from build123d import *

# Parameters (mm, degrees)
SKETCH_8_R          = 8
SKETCH_8_R_2        = 1.5
SKETCH_8_R_3        = 1.55
SKETCH_8_R_4        = 2.05
EXTRUDE_2522_DEPTH  = 3
FILLET_27_R         = 6
FILLET_30_R         = 3
FILLET_31_R         = 2
SKETCH_9_R          = 2.05
CUT_EXTRUDE_1_DEPTH = 172.249087589


with BuildPart() as part:
    # Эскиз8 → Extrude 2522 (new body)
    with BuildSketch(Plane.XY):
        with BuildLine():
            Line((38.676576093, 1), (169, 1))
            Line((169, 1), (169, -15))
            Line((169, -15), (90, -15))
            Line((90, -15), (12, -15))
            Line((12, -15), (10, -17))
            Line((10, -17), (4.230786919, -17))
            ThreePointArc((4.230786919, -17), (0, -17.231764199), (-4.230786919, -17))
            Line((-4.230786919, -17), (-10, -17))
            Line((-10, -17), (-12, -15))
            Line((-12, -15), (-90, -15))
            Line((-90, -15), (-169, -15))
            Line((-169, -15), (-169, 1))
            Line((-169, 1), (-38.676576093, 1))
            ThreePointArc((-38.676576093, 1), (-20.275683212, 5.483705976), (-6, 17.929642941))
            Line((-6, 17.929642941), (-6, 27.5))
            Line((-6, 27.5), (6, 27.5))
            Line((6, 27.5), (6, 17.929642941))
            ThreePointArc((6, 17.929642941), (20.275683212, 5.483705976), (38.676576093, 1))
        make_face()
        Circle(SKETCH_8_R, mode=Mode.SUBTRACT)
        with Locations((0, -12.5)):
            Circle(SKETCH_8_R_2, mode=Mode.SUBTRACT)
        with Locations((163, -7)):
            Circle(SKETCH_8_R_3, mode=Mode.SUBTRACT)
        with Locations((111, -7)):
            Circle(SKETCH_8_R_3, mode=Mode.SUBTRACT)
        with Locations((0, 21.5)):
            Circle(SKETCH_8_R_4, mode=Mode.SUBTRACT)
        with Locations((127, -7)):
            Circle(SKETCH_8_R_3, mode=Mode.SUBTRACT)
        with Locations((-10.825317547, 6.25)):
            Circle(SKETCH_8_R_2, mode=Mode.SUBTRACT)
        with Locations((10.825317547, 6.25)):
            Circle(SKETCH_8_R_2, mode=Mode.SUBTRACT)
        with Locations(Location((-127, -7, 0), (0, 0, 180))):
            Circle(SKETCH_8_R_3, mode=Mode.SUBTRACT)
        with Locations(Location((-111, -7, 0), (0, 0, 180))):
            Circle(SKETCH_8_R_3, mode=Mode.SUBTRACT)
        with Locations(Location((-163, -7, 0), (0, 0, 180))):
            Circle(SKETCH_8_R_3, mode=Mode.SUBTRACT)
    extrude(amount=EXTRUDE_2522_DEPTH)

    # Скругление27
    fillet_27_edges = [part.edges().sort_by_distance(p)[0] for p in [
        (-6, 27.5, 1.5),
        (6, 27.5, 1.5),
    ]]
    fillet(fillet_27_edges, radius=FILLET_27_R - 0.0001)  # a hair under: the kernel refuses the full size

    # Скругление30
    fillet_30_edges = [part.edges().sort_by_distance(p)[0] for p in [
        (12, -15, 1.5),
        (10, -17, 1.5),
        (-10, -17, 1.5),
        (-12, -15, 1.5),
    ]]
    fillet(fillet_30_edges, radius=FILLET_30_R)

    # Скругление31
    fillet_31_edges = [part.edges().sort_by_distance(p)[0] for p in [
        (169, 1, 1.5),
        (169, -15, 1.5),
        (-169, -15, 1.5),
        (-169, 1, 1.5),
    ]]
    fillet(fillet_31_edges, radius=FILLET_31_R)

    # Эскиз9 → Вырез-Вытянуть1 (cut, through all)
    with BuildSketch(Plane.XY.offset(3)):
        with Locations((-65, -7)):
            Circle(SKETCH_9_R)
        with Locations(Location((65, -7, 0), (0, 0, 180))):
            Circle(SKETCH_9_R)
    extrude(amount=-CUT_EXTRUDE_1_DEPTH, mode=Mode.SUBTRACT)


solid = part.part
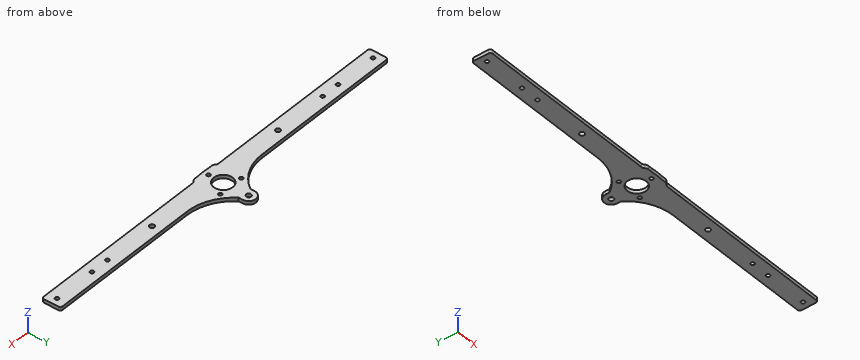
Geometry: final body of the model. Coordinates: model frame, mm. Coordinates: 2 decimals unless noted, no trailing zeros. Order: outer loops, then holes, each group sorted by start corner. A loop starts at its lowest first (then second) coordinate and runs counter-clockwise, first axis right, second up.
1) First-contact query: P1, Ø1.5, axis at y = 19.5, z = 2, coming from the -X side; P2, Ø0.9, axis at x = 6, z = 1, coming from the -Y side; P3, Ø1.5, axis at x = 79, z = 2, coming from the -Y side. Flat tips, straight axial feed; report the tip coordinate or a pass-through.
Result sheet:
P1: stops at x = -6
P2: stops at y = -17
P3: stops at y = -15
2) Section B-B (z = 0.8). Give the number of separate pieces and of enclosed holes in the cut face, then the cut area to 3 significant figures.
Result sheet:
separate pieces: 1
enclosed holes: 13
area: 5,780 mm2
3) Ray query, probe 1 along Y at (x, z) = (-65, 0.75); probe 2 along Y at (x, z) = (0, 1.35); probe 3 along Y at (x, z) = (-127, 1.2). Return the intervals inside material, ascending.
Result sheet:
probe 1: y = -15 to -9.05, -4.95 to 1
probe 2: y = -17.23 to -14, -11 to -8, 8 to 19.45, 23.55 to 27.5
probe 3: y = -15 to -8.55, -5.45 to 1
4) Section A-A (x = 70). Return loops of the section in (y, z).
Result sheet:
outline: (-15, 0) - (1, 0) - (1, 3) - (-15, 3) - close
5) Section C-C (y = 14.5). Return loops of the section in (x, z).
Result sheet:
outline: (-8.71, 0) - (8.71, 0) - (8.71, 3) - (-8.71, 3) - close
